Autodesk Inventor part; units mm, degrees
ref_plane "YZ Plane" through (0, 0, 0) normal (1, 0, 0) x (0, 1, 0)
ref_plane "XZ Plane" through (0, 0, 0) normal (0, 1, 0) x (-1, 0, 0)
ref_plane "XY Plane" through (0, 0, 0) normal (0, 0, 1) x (1, 0, 0)
sketch "Sketch1" plane through (0, 0, 0) normal (0, 1, 0) x (-1, 0, 0)
  line L0 (-7.5, 25) -> (7.5, 25)
  line L1 (7.5, 25) -> (7.5, -25)
  line L2 (7.5, -25) -> (-7.5, -25)
  line L3 (-7.5, -25) -> (-7.5, 25)
  line L4 (-7.5, 25) -> (7.5, -25) construction
  line L5 (7.5, 25) -> (-7.5, -25) construction
  line L6 (0.5, -19) -> (-0.5, -19)
  line L7 (-0.5, 19) -> (0.5, 19)
  circle A0 centre (0, 19) radius 1.5
  circle A1 centre (0, -19) radius 1.5
  line L8 (7.5, -25) -> (-7.5, -25)
  line L9 (-7.5, -25) -> (-7.5, -23)
  line L10 (-7.5, -23) -> (7.5, -23)
  line L11 (7.5, -23) -> (7.5, -25)
  line L12 (7.5, 25) -> (-7.5, 25)
  line L13 (-7.5, 25) -> (-7.5, 23)
  line L14 (-7.5, 23) -> (7.5, 23)
  line L15 (7.5, 23) -> (7.5, 25)
  point P0 (0, 0)
  point P1 (0, 0)
  dimension "d0" = 15
  dimension "d1" = 50
  dimension "d2" = 1
  dimension "d3" = 38
  dimension "d4" = 3
  dimension "d5" = 3
  dimension "d6" = 15
  dimension "d7" = 2
  dimension "d8" = 15
  dimension "d9" = 2
extrude "Extrusion1" add sketch "Sketch1" along normal blind 2 contours L14 L1 L10 L3
extrude "Extrusion2" add sketch "Sketch1" along normal blind 25 contours L0 L1 L14 L3 | L10 L1 L2 L3
sketch "Sketch2" plane through (-7.5, 0, 25) normal (0, 0, 1) x (1, 0, 0)
  line L0 (7.5, 0) -> (7.5, 18)
  line L1 (7.5, 0) -> (25.5, 0) construction
  circle A0 centre (7.5, 18) radius 4
  dimension "d14" = 18
  dimension "d15" = 90
  dimension "d16" = 8
extrude "Extrusion3" cut sketch "Sketch2" against normal blind 50
fillet "Fillet1" radius 4 4 edges at (-7.5, 25, -24) (7.5, 25, -24) (-7.5, 25, 24) (7.5, 25, 24)
properties part number "senzor_drzak"
Read the model definition and answer for the solid it produces. Units are mm, in the model's axes. A direction names the side the tool comes from. Round coordinates to 2 decimals unless told otherwise and drop trailing zeros. Write each loop counter-clockwise with the first axis right and the second up, starting at its lowest first coordinate (ties: lowest second). Pieces come first, ordered by that corner, then holes. Notation, with made-up numbers: (42, 39) - (53, 39) arc R12 cw to (53, 47) - close; hole circle Ø5 at (10.5, 72.5). An arc over 180 degrees is marked (long way). One line per question, with ' | ' between items. Start each with the question number.
1. For a pull along X with two mould halves and no side action, classify faces 1 (the face through (0, 2, 0)), 2 (the face through (-7.5, 1, 0)), 3 (the face through (0.195, 0.986, -20.487)), 4 (the face through (-0.521, 21.966, 24.014)) as +X half, -X half, draft (parallel to the pull), parting line (faces both ways), or undercut.
2. Find the intervals of material crossed by probe 1 along X at (y, z) = (18, -24.1); probe 2 along Z at (x, y) = (0, 1); probe 3 along Z at (x, y) = (1, 4.75), in increasing order. Write a range as [from, to].
3. Section C-C (y = 18) is taken. Determine the outline of the cut face in (x, z).
4. Section A-A (y = 11.25) is taken. Determine the outline of the cut face in (x, z), and give its area (3 significant figures).
5. For faces 5 (the face through (0, 0, 0)), 6 (the face through (0, 13, -23)), determine the directions among +Z, -Z, +X, -X, +Y, -Y from which every point of the face is accessible in a straight line to the end or side of a thin tool.
6. Section D-D (x = 0) is taken. Determine the outline of the cut face in (y, z).
7. Section B-B (z = -19) is taken. Determine the outline of the cut face in (x, y).
8. Each of these flat-tipped pins is pushed along its axis until it touches: pin 1 (5 mm diameter, centred on x = -1, z = -17.5, fed in from +Y); pin 2 (2.5 mm diameter, centred on x = 0, z = 19, fed in from -Y). Where does it stop, or does it pass through?
Filled in:
1) face 1: draft | face 2: -X half | face 3: undercut | face 4: undercut
2) probe 1: [-7.5, -4], [4, 7.5] | probe 2: [-25, -20.5], [-17.5, 17.5], [20.5, 25] | probe 3: [-25, -23], [23, 25]
3) outline: (-7.5, -25) - (-4, -25) - (-4, -23) - (-7.5, -23) - close; (-7.5, 23) - (-4, 23) - (-4, 25) - (-7.5, 25) - close; (4, -25) - (7.5, -25) - (7.5, -23) - (4, -23) - close; (4, 23) - (7.5, 23) - (7.5, 25) - (4, 25) - close
4) outline: (-7.5, -25) - (7.5, -25) - (7.5, -23) - (-7.5, -23) - close; (-7.5, 23) - (7.5, 23) - (7.5, 25) - (-7.5, 25) - close | area: 60.0 mm²
5) face 5: +Z, -Z, +X, -X, -Y | face 6: +X, -X, +Y
6) outline: (0, -25) - (14, -25) - (14, -23) - (2, -23) - (2, -20.5) - (0, -20.5) - close; (0, -17.5) - (2, -17.5) - (2, 17.5) - (0, 17.5) - close; (0, 20.5) - (2, 20.5) - (2, 23) - (14, 23) - (14, 25) - (0, 25) - close; (22, -25) - (25, -25) - (25, -23) - (22, -23) - close; (22, 23) - (25, 23) - (25, 25) - (22, 25) - close
7) outline: (-7.5, 0) - (-1.5, 0) - (-1.5, 2) - (-7.5, 2) - close; (1.5, 0) - (7.5, 0) - (7.5, 2) - (1.5, 2) - close
8) pin 1: y = 2 | pin 2: through
